from build123d import *

# Parameters (mm, degrees)
F0_W      = 80
F0_H      = 36.3
F1_DEPTH  = 4.5
F2_R      = 4
F3_W      = 63
F3_H      = 30.3
F4_DEPTH  = 3.5
F5_W      = 5
F5_H      = 16.5
F5_W_2    = 3.5
F5_H_2    = 6.5
F6_DEPTH  = 4.501
F7_W      = 2
F7_H      = 18
F8_DEPTH  = 1
F10_DEPTH = 3
F11_R     = 1.6
F12_DEPTH = 4.501
F13_R     = 3
F14_DEPTH = 3
F15_W     = 5
F15_H     = 11
F16_DEPTH = 0.6


with BuildPart() as f1:
    # F0 (on Top) → F1 (new body)
    with BuildSketch(Plane.XY):
        with Locations((37, 15.15)):
            Rectangle(F0_W, F0_H)
    extrude(amount=F1_DEPTH)

    # F2
    f2_edges = [f1.edges().sort_by_distance(p)[0] for p in [
        (-3, -3, 2.25),
        (77, -3, 2.25),
        (77, 33.3, 2.25),
        (-3, 33.3, 2.25),
    ]]
    fillet(f2_edges, radius=F2_R)

    # F3 (on face) → F4 (cut)
    with BuildSketch(Plane.XY.offset(4.5)):
        with Locations((31.5, 15.15)):
            Rectangle(F3_W, F3_H)
    extrude(amount=-F4_DEPTH, mode=Mode.SUBTRACT)

    # F5 (on face) → F6 (cut, through all)
    with BuildSketch(Plane.XY.offset(4.5)):
        with Locations((2.5, 15.15)):
            Rectangle(F5_W, F5_H)
        with Locations((38, 24.55)):
            Rectangle(F5_W_2, F5_H_2)
    extrude(amount=-F6_DEPTH, mode=Mode.SUBTRACT)

    # F7 (on face) → F8 (cut)
    with BuildSketch(Plane.XY.offset(4.5)):
        with Locations((64, 13)):
            Rectangle(F7_W, F7_H)
    extrude(amount=-F8_DEPTH, mode=Mode.SUBTRACT)

    # F9 (on face) → F10 (join)
    with BuildSketch(Plane.XY.offset(1)):
        with BuildLine():
            Line((8, 30.3), (0, 30.3))
            Line((0, 30.3), (0, 23.4))
            Line((0, 23.4), (5, 23.4))
            ThreePointArc((5, 23.4), (7.12132, 24.27868), (8, 26.4))
            Line((8, 26.4), (8, 30.3))
        make_face()
        with BuildLine():
            Line((5, 6.9), (0, 6.9))
            Line((0, 6.9), (0, 0))
            Line((0, 0), (8, 0))
            Line((8, 0), (8, 3.9))
            ThreePointArc((8, 3.9), (7.12132, 6.02132), (5, 6.9))
        make_face()
    extrude(amount=F10_DEPTH)

    # F11 (on face) → F12 (cut, through all)
    with BuildSketch(Plane.XY.offset(4.5)):
        with Locations((4.35, 4.35)):
            Circle(F11_R)
        with Locations((4.35, 25.95)):
            Circle(F11_R)
        with Locations((69.65, 25.95)):
            Circle(F11_R)
        with Locations((69.65, 4.35)):
            Circle(F11_R)
    extrude(amount=-F12_DEPTH, mode=Mode.SUBTRACT)

    # F13 (on face) → F14 (cut)
    with BuildSketch(Plane(origin=(0, 0, 0), x_dir=(1, 0, 0), z_dir=(0, 0, -1))):
        with Locations((69.65, -25.95)):
            Circle(F13_R)
        with Locations((69.65, -4.35)):
            Circle(F13_R)
        with BuildLine():
            ThreePointArc((4.35, -28.95), (6.47132, -28.07132), (7.35, -25.95))
            ThreePointArc((7.35, -25.95), (2.22868, -23.82868), (4.35, -28.95))
        make_face()
        with Locations((4.35, -4.35)):
            Circle(F13_R)
    extrude(amount=-F14_DEPTH, mode=Mode.SUBTRACT)

    # F15 (on face) → F16 (cut)
    with BuildSketch(Plane.XY.offset(1)):
        with Locations((22.5, 23.05)):
            Rectangle(F15_W, F15_H)
    extrude(amount=-F16_DEPTH, mode=Mode.SUBTRACT)


solid = f1.part
Could you check a few things on this model? Use its own coordinates, in mm. A direction names the side the tool comes from. Round coordinates to 2 decimals unless told otherwise and drop trailing zeros. Order: outer loops, then holes, each group sorted by start corner. A loop starts at its lowest first (then second) coordinate and runs counter-clockwise, first axis right, second up.
Q1. I'm going to push flat-ended pins straight in: P1, Ø2.5, axis at x = 69.65, y = 4.35, coming from the +Z side; P2, Ø2, axis at x = 5, y = 25.5, coming from the +Z side; P3, Ø15, axis at x = 38, y = 20, coming from the +Z side. Where does each tip first touch, or does it pass through?
Geometry says:
P1: passes through
P2: stops at z = 4
P3: stops at z = 1
Q2. Imagine slicing it at B-B, the plane x = 69.65. List the corners of the cut face in (y, z) for me, then the cut area to 3 significant figures.
Geometry says:
outline: (-3, 0) - (1.35, 0) - (1.35, 3) - (2.75, 3) - (2.75, 4.5) - (-3, 4.5) - close; (5.95, 3) - (7.35, 3) - (7.35, 0) - (22.95, 0) - (22.95, 3) - (24.35, 3) - (24.35, 4.5) - (5.95, 4.5) - close; (27.55, 3) - (28.95, 3) - (28.95, 0) - (33.3, 0) - (33.3, 4.5) - (27.55, 4.5) - close
area: 118 mm2
Q3. Thinking about a two-plate mould opening in X: for faces 4 (the face through (-1.859, -1.797, 2.282)), 5 (the face through (71, 6, 3)), 6 (the face through (75.859, 32.097, 2.282)), 7 (the face through (31, 30.3, 3)), which applies, released by +X, released by -X, zero draft, split by the parting line, or undercut?
Geometry says:
face 4: released by -X
face 5: undercut
face 6: released by +X
face 7: undercut
Q4. Imagine slicing it at C-C, the plane x = 51.5. List the corners of the cut face in (y, z) for me.
Geometry says:
outline: (-3, 0) - (33.3, 0) - (33.3, 4.5) - (30.3, 4.5) - (30.3, 1) - (0, 1) - (0, 4.5) - (-3, 4.5) - close
Q5. Please list where these lines run through material, in increasing order: probe 1 along Y at (x, z) = (4.35, 3.65); probe 2 along Y at (x, z) = (69.65, 2.35); probe 3 along Y at (x, z) = (69.65, 4.1).
Geometry says:
probe 1: y = -3 to 2.75, 5.95 to 6.9, 23.4 to 24.35, 27.55 to 33.3
probe 2: y = -3 to 1.35, 7.35 to 22.95, 28.95 to 33.3
probe 3: y = -3 to 2.75, 5.95 to 24.35, 27.55 to 33.3
Q6. Imagine slicing it at A-A, the plane y = 9.5. List the corners of the cut face in (x, z) for me.
Geometry says:
outline: (-3, 0) - (0, 0) - (0, 4.5) - (-3, 4.5) - close; (5, 0) - (77, 0) - (77, 4.5) - (65, 4.5) - (65, 3.5) - (63, 3.5) - (63, 1) - (5, 1) - close
Q7. Which directions (+Z, -Z, +X, -X, +Y, -Y) give clear straight access to the entire face, cutting with the end or side of a thin tool? Please do faces 1 (the face through (70.9, 27.2, 3)), 2 (the face through (-3, 15, 2)), 3 (the face through (64, 13, 3.5)).
Geometry says:
face 1: -Z
face 2: +Z, -Z, -X, +Y, -Y
face 3: +Z
Q8. Imagine slicing it at D-D, the plane x = 3.5. List the corners of the cut face in (y, z) for me.
Geometry says:
outline: (-3, 0) - (1.47, 0) - (1.47, 3) - (2.99, 3) - (2.99, 4) - (0, 4) - (0, 4.5) - (-3, 4.5) - close; (5.71, 3) - (6.9, 3) - (6.9, 4) - (5.71, 4) - close; (23.4, 3) - (24.59, 3) - (24.59, 4) - (23.4, 4) - close; (27.31, 3) - (28.83, 3) - (28.83, 0) - (33.3, 0) - (33.3, 4.5) - (30.3, 4.5) - (30.3, 4) - (27.31, 4) - close
